Can you work these out from the model? Positions are in its coordinate system, mm. A direction names the side the tool comes from. Coordinates: 2 decimals unless noted, no trailing zeros. Order: outer loops, then holes, each group sorted by start corner. A loop starts at its lowest first (then second) coordinate and runs counter-clockwise, first axis right, second up. Notation, with made-up numbers: (24, 37) -> (28, 37) arc R31 cw to (28, 67) -> close; hole circle Ø10 at (68, 45.25). An arc over 180 degrees is marked (long way). Answer in a Markdown table with one row per item.
```python
from build123d import *

# Parameters (mm, degrees)
F1_DEPTH  = 6.35
F2_W      = 215.9
F2_H      = 76.2
F3_DEPTH  = 6.35
F4_W      = 196.85
F4_H      = 76.2
F5_DEPTH  = 6.35
F7_DEPTH  = 6.35
F8_W      = 6.35
F8_H      = 215.9
F9_DEPTH  = 76.2
F10_W     = 6.35
F10_H     = 25.4
F11_DEPTH = 12.7


with BuildPart() as f1:
    # F0 (on Front) → F1 (new body)
    with BuildSketch(Plane.XZ):
        Polygon((0, 76.2), (0, 0), (25.4, 0), (25.4, 50.8), (63.5, 50.8), (63.5, 0), (88.9, 0), (88.9, 50.8), (127, 50.8), (127, 0), (152.4, 0), (152.4, 50.8), (190.5, 50.8), (190.5, 0), (215.9, 0), (215.9, 50.8), (254, 50.8), (254, 0), (279.4, 0), (279.4, 41.275), (317.5, 41.275), (317.5, 0), (342.9, 0), (342.9, 127), (266.7, 127), (266.7, 76.2), align=None)
    extrude(amount=F1_DEPTH)

    # F2 (on Right) → F3 (join)
    with BuildSketch(Plane.YZ):
        with Locations((107.95, 38.1)):
            Rectangle(F2_W, F2_H)
    extrude(amount=F3_DEPTH)

    # F4 (on face) → F5 (join)
    with BuildSketch(Plane(origin=(0, 215.9, 0), x_dir=(-1, 0, 0), z_dir=(0, 1, 0))):
        with Locations((-98.425, 38.1)):
            Rectangle(F4_W, F4_H)
    extrude(amount=F5_DEPTH)

    # F6 (on face) → F7 (join)
    with BuildSketch(Plane.YZ.offset(196.85)):
        Polygon((222.25, 0), (222.25, 76.2), (133.35, 76.2), (133.35, 0), (158.75, 0), (158.75, 50.8), (196.85, 50.8), (196.85, 0), align=None)
    extrude(amount=F7_DEPTH)

    # F8 (on face) → F9 (join)
    with BuildSketch(Plane.XY.offset(76.2)):
        with Locations((76.2, 107.95)):
            Rectangle(F8_W, F8_H)
    extrude(amount=-F9_DEPTH)

    # F10 (on face) → F11 (cut)
    with BuildSketch(Plane.YZ.offset(79.375)):
        with Locations((9.525, 12.7)):
            Rectangle(F10_W, F10_H)
    extrude(amount=-F11_DEPTH, mode=Mode.SUBTRACT)


solid = f1.part
```
(1) Will these pins go through, and if not, where does the flat tip stop? pin 1 Ø12 at (x, z) = (182, 40.5) entering from -Y; pin 2 Ø7 at (x, y) = (303, -5) entering from -Z (3 decimals); pin 3 Ø1.5 at (x, z) = (284.5, 53) entering from +Y.
Response values:
| item | result |
|---|---|
| pin 1 | y = 215.9 |
| pin 2 | z = 41.275 |
| pin 3 | y = 0 |
(2) Suppose I cut it at C-C (x = 148). Please give me the cut outline in (y, z), and give its area (3 significant figures).
Response values:
| item | result |
|---|---|
| outline | (-6.35, 0) -> (0, 0) -> (0, 76.2) -> (-6.35, 76.2) -> close; (215.9, 0) -> (222.25, 0) -> (222.25, 76.2) -> (215.9, 76.2) -> close |
| area | 968 mm2 |
(3) I need wall thicknesses on line 1 (X direction, y = 147.5, z = 29.5) (3 decimals); line 2 (Y direction, x = 141, z = 24.5); line 3 (X direction, y = 40, z = 41.5) (3 decimals). Which ranges of each line are inside material? Lowest first, please. Write a range as [from, to].
Response values:
| item | result |
|---|---|
| line 1 | [0, 6.35], [73.025, 79.375], [196.85, 203.2] |
| line 2 | [-6.35, 0], [215.9, 222.25] |
| line 3 | [0, 6.35], [73.025, 79.375] |
(4) Suppose I cut it at D-D (y = 83.5). Please give me the cut outline in (x, z) (3 decimals), and give its area (3 significant figures).
Response values:
| item | result |
|---|---|
| outline | (0, 0) -> (6.35, 0) -> (6.35, 76.2) -> (0, 76.2) -> close; (73.025, 0) -> (79.375, 0) -> (79.375, 76.2) -> (73.025, 76.2) -> close |
| area | 968 mm2 |
(5) Suppose I cut it at A-A (z = 57.5). Please give me the cut outline in (x, y) (3 decimals), and give its area (3 significant figures).
Response values:
| item | result |
|---|---|
| outline | (0, -6.35) -> (342.9, -6.35) -> (342.9, 0) -> (79.375, 0) -> (79.375, 215.9) -> (196.85, 215.9) -> (196.85, 133.35) -> (203.2, 133.35) -> (203.2, 222.25) -> (0, 222.25) -> close; hole (6.35, 0) -> (73.025, 0) -> (73.025, 215.9) -> (6.35, 215.9) -> close |
| area | 6,730 mm2 |
(6) We'd pull the mould along Y, two halves only. Please class faces 1 (the flat face through (73.025, 106, 39)), 2 (the flat face through (76, -2, 0)), 3 (the flat face through (196.85, 174, 56)), 4 (the flat face through (207, -6.35, 50)): +Y half, -Y half, draft (parallel to the pull), parting line (faces both ways), or undercut.
Response values:
| item | result |
|---|---|
| face 1 | undercut |
| face 2 | draft |
| face 3 | undercut |
| face 4 | -Y half |
(7) On a 3-axis mill with a long thin cutter (end or side, diameter ignored), from which of +Z, -Z, +X, -X, +Y, -Y can I reach the whole of each face in a straight line? I mean faces 5 (the flat face through (239, 0, 64)), 6 (the flat face through (73.5, 108.5, 76.2)), 7 (the flat face through (32, 0, 56)). Say none if no direction works.
Response values:
| item | result |
|---|---|
| face 5 | +Z, -Z, +X |
| face 6 | +Z, -X, +Y, -Y |
| face 7 | +Z, -Z |
(8) Suppose I cut it at B-B (y = 176.5). Please give me the cut outline in (x, z) (3 decimals), and give its area (3 significant figures).
Response values:
| item | result |
|---|---|
| outline | (0, 0) -> (6.35, 0) -> (6.35, 76.2) -> (0, 76.2) -> close; (73.025, 0) -> (79.375, 0) -> (79.375, 76.2) -> (73.025, 76.2) -> close; (196.85, 50.8) -> (203.2, 50.8) -> (203.2, 76.2) -> (196.85, 76.2) -> close |
| area | 1,130 mm2 |
